from build123d import *

# Parameters (mm, degrees)
SKETCH_1_W                = 127
SKETCH_1_H                = 65
SKETCH_1_W_2              = 100
SKETCH_1_H_2              = 45
SKETCH_5_W                = 50
SKETCH_5_H                = 65
EXTRUDE_1_DEPTH           = 4
SKETCH_6_W                = 50
SKETCH_6_H                = 65
EXTRUDE_2_DEPTH           = 4
CHAMFER_1_SIZE            = 4
SKETCH_9_W                = 44
SKETCH_9_H                = 45
CUT_EXTRUDE_1_DEPTH       = 15
SKETCH_10_W               = 44
SKETCH_10_H               = 45
CUT_EXTRUDE_2_DEPTH       = 15
HOLE_WIZARD_6_0_6_1_D     = 6
HOLE_WIZARD_6_0_6_2_D     = 6
HOLE_WIZARD_6_0_6_2_DEPTH = 65
HOLE_WIZARD_6_0_6_3_D     = 6
HOLE_WIZARD_6_0_6_3_DEPTH = 10
HOLE_WIZARD_6_0_6_4_D     = 6
HOLE_WIZARD_6_0_6_4_DEPTH = 10


with BuildPart() as part:
    # 掃出1: sweep along a path in 草圖2
    with BuildLine(Plane(origin=(0, 0, 0), x_dir=(0, 0, -1), z_dir=(1, 0, 0))) as sweep_1_path:
        Line((0, 0), (2150, 0))
        ThreePointArc((2150, 0), (2350, 200), (2150, 400))
        Line((2150, 400), (2050, 400))
    # 草圖1 → 掃出1 (sweep)
    with BuildSketch(Plane.XY):
        Rectangle(SKETCH_1_W, SKETCH_1_H)
        Rectangle(SKETCH_1_W_2, SKETCH_1_H_2, mode=Mode.SUBTRACT)
    sweep(path=sweep_1_path.line)

    # 草圖5 → 伸長1 (add)
    with BuildSketch(Plane(origin=(63.5, 0, 0), x_dir=(0, 0, -1), z_dir=(1, 0, 0))):
        with Locations((25, 0)):
            Rectangle(SKETCH_5_W, SKETCH_5_H)
        with Locations((2075, 400)):
            Rectangle(SKETCH_5_W, SKETCH_5_H)
    extrude(amount=EXTRUDE_1_DEPTH)

    # 草圖6 → 伸長2 (add)
    with BuildSketch(Plane.ZY.offset(63.5)):
        with Locations((-2075, 400)):
            Rectangle(SKETCH_6_W, SKETCH_6_H)
        with Locations((-25, 0)):
            Rectangle(SKETCH_6_W, SKETCH_6_H)
    extrude(amount=EXTRUDE_2_DEPTH)

    # 導角1
    chamfer_1_edges = [part.edges().sort_by_distance(p)[0] for p in [
        (63.5, 0, -50),
        (63.5, 400, -2100),
        (-63.5, 400, -2100),
        (-63.5, 0, -50),
    ]]
    chamfer(chamfer_1_edges, length=CHAMFER_1_SIZE - 0.0001)  # a hair under: the kernel refuses the full size

    # 草圖9 → 除料-伸長1 (cut)
    with BuildSketch(Plane(origin=(67.5, 0, 0), x_dir=(0, 0, -1), z_dir=(1, 0, 0))):
        with Locations((32, 0)):
            Rectangle(SKETCH_9_W, SKETCH_9_H)
        with Locations((2082, 400)):
            Rectangle(SKETCH_9_W, SKETCH_9_H)
    extrude(amount=-CUT_EXTRUDE_1_DEPTH, mode=Mode.SUBTRACT)

    # 草圖10 → 除料-伸長2 (cut)
    with BuildSketch(Plane.ZY.offset(67.5)):
        with Locations((-2082, 400)):
            Rectangle(SKETCH_10_W, SKETCH_10_H)
        with Locations((-32, 0)):
            Rectangle(SKETCH_10_W, SKETCH_10_H)
    extrude(amount=-CUT_EXTRUDE_2_DEPTH, mode=Mode.SUBTRACT)

    # Ø6.0 (6) 直徑孔1 (through all)
    with Locations(Plane(origin=(0, 32.5, 0), x_dir=(-1, 0, 0), z_dir=(0, 1, 0))):
        with Locations((59, -40), (59, -16), (-59, -16), (-59, -40)):
            Hole(HOLE_WIZARD_6_0_6_1_D / 2)

    # Ø6.0 (6) 直徑孔2
    with Locations(Plane(origin=(0, 432.5, 0), x_dir=(-1, 0, 0), z_dir=(0, 1, 0))):
        with Locations((59, -2090), (59, -2066), (-59, -2090), (-59, -2066)):
            Hole(HOLE_WIZARD_6_0_6_2_D / 2, depth=HOLE_WIZARD_6_0_6_2_DEPTH)

    # Ø6.0 (6) 直徑孔3
    with Locations(Plane.XY):
        with Locations((-59, 12), (-59, -12), (59, 12), (59, -12)):
            Hole(HOLE_WIZARD_6_0_6_3_D / 2, depth=HOLE_WIZARD_6_0_6_3_DEPTH)

    # Ø6.0 (6) 直徑孔4
    with Locations(Plane.XY.offset(-2050)):
        with Locations((-59, 412), (-59, 388), (59, 412), (59, 388)):
            Hole(HOLE_WIZARD_6_0_6_4_D / 2, depth=HOLE_WIZARD_6_0_6_4_DEPTH)


solid = part.part
Source: CAD feature listing. Evaluate the final solid. Frame: model axes, mm. A direction names the side the tool comes from. Coordinates: 2 decimals unless noted, no trailing zeros. Loops run counter-clockwise (first coordinate to the right, second up) from the corner with the lowest first, then second, coordinate; pieces in that order, holes last. Notation, with made-up numbers: (10, -12) - (47, -12) arc R29 cw to (47, 19) - close; hole circle Ø11 at (80.5, -14.5). An arc over 180 degrees is marked (long way). Return JSON: item names as keys, results as strings.
Q1. Mould query, pull axis X, two halves, no side actions, for faces 6 (the flat face through (63.5, 27, -1396)), 7 (the cylindrical face through (-0.89, 196.32, -2317.46)), 8 (the cylindrical face through (0.7, 196.097, -2327.457)), 9 (the flat face through (-52.5, 0, -32)). Classes: released by +X, released by -X, zero draft, split by the parting line, or undercut.
Results:
{"face 6": "released by +X", "face 7": "zero draft", "face 8": "undercut", "face 9": "released by -X"}
Q2. Section A-A, the plane x = -0.5. Return loops of the section in (y, z).
Results:
{"outline": "(-32.5, -2150) arc R232.5 ccw to (432.5, -2150) - (432.5, -2050) - (422.5, -2050) - (422.5, -2150) arc R222.5 cw to (-22.5, -2150) - (-22.5, 0) - (-32.5, 0) - close; (22.5, -2150) arc R177.5 ccw to (377.5, -2150) - (377.5, -2050) - (367.5, -2050) - (367.5, -2150) arc R167.5 cw to (32.5, -2150) - (32.5, 0) - (22.5, 0) - close"}
Q3. Material intervals for line 1 along Y through (x, z) = (-59, -2056.25); line 2 along X through (y, z) = (373, -2066); line 3 along Y through (x, z) = (-59, -4), sorted ascending.
Results:
{"line 1": "-32.5 to 32.5, 367.5 to 385, 391 to 409, 415 to 432.5", "line 2": "-67.5 to -62, -56 to 56, 62 to 67.5", "line 3": "-32.5 to -15, -9 to 9, 15 to 32.5"}
Q4. Section C-C, the plane z = -1985.5. Return loops of the section in (x, y).
Results:
{"outline": "(-63.5, -32.5) - (63.5, -32.5) - (63.5, 32.5) - (-63.5, 32.5) - close; hole (-50, -22.5) - (50, -22.5) - (50, 22.5) - (-50, 22.5) - close"}
Q5. Access query for faces 1 (the flat face through (52.5, 400, -2082)), 2 (the flat face through (-50, 18, -1368)), 3 (the flat face through (1, 367.5, -2101)), 4 (the flat face through (-52.5, 400, -2082)), 5 (the flat face through (-1, 22.5, -1090)). Directions: +Z, -Z, +X, -X, +Y, -Y. A direction counts if a zero-diameter tool reaches every point of the face in a straight line with its end or side. Return the directions, or none.
Results:
{"face 1": "+X", "face 2": "none", "face 3": "+Z, +X, -X", "face 4": "-X", "face 5": "+Z"}
Q6. Contact query for flat-ended pins moving along their axis: P1, Ø2, axis at x = -16.5, z = -622, coming from the +Y side; P2, Ø5, axis at x = -59, y = -12, coming from the +Z side; P3, Ø10, axis at x = 22, y = 149.5, coming from the +Z side. Output: stop coordinate, or through.
Results:
{"P1": "y = 32.5", "P2": "z = -54", "P3": "z = -2308.04"}
Q7. Section B-B, the plane y = 200. Return loops of the section in (x, z).
Results:
{"outline": "(-63.5, -2382.5) - (63.5, -2382.5) - (63.5, -2317.5) - (-63.5, -2317.5) - close; hole (-50, -2372.5) - (50, -2372.5) - (50, -2327.5) - (-50, -2327.5) - close"}
